```python
from build123d import *

# Parameters (mm, degrees)
SKETCH_1_W          = 17
SKETCH_1_H          = 17
EXTRUDE_1_DEPTH     = 70
SKETCH_2_W          = 12
SKETCH_2_H          = 12
CUT_EXTRUDE_1_DEPTH = 66
SKETCH_3_R          = 1.5
CUT_EXTRUDE_2_DEPTH = 8


with BuildPart() as part:
    # 草图1 → 凸台-拉伸1 (new body)
    with BuildSketch(Plane(origin=(0, 0, 0), x_dir=(1, 0, 0), z_dir=(0, 1, 0))):
        with Locations((8.5, -8.5)):
            Rectangle(SKETCH_1_W, SKETCH_1_H)
    extrude(amount=EXTRUDE_1_DEPTH)

    # 草图2 → 切除-拉伸1 (cut)
    with BuildSketch(Plane(origin=(0, 70, 0), x_dir=(1, 0, 0), z_dir=(0, 1, 0))):
        with Locations((6, -6)):
            Rectangle(SKETCH_2_W, SKETCH_2_H)
    extrude(amount=-CUT_EXTRUDE_1_DEPTH, mode=Mode.SUBTRACT)

    # 草图3 → 切除-拉伸2 (cut)
    with BuildSketch(Plane(origin=(0, 0, 0), x_dir=(-1, 0, 0), z_dir=(0, -1, 0))):
        with Locations(Location((-9.574531369, -2.425468631, 0), (0, 0, 90))):
            Circle(SKETCH_3_R)
        with Locations(Location((-2.425468631, -2.425468631, 0), (0, 0, 90))):
            Circle(SKETCH_3_R)
        with Locations(Location((-9.574531369, -9.574531369, 0), (0, 0, 90))):
            Circle(SKETCH_3_R)
        with Locations(Location((-2.425468631, -9.574531369, 0), (0, 0, 90))):
            Circle(SKETCH_3_R)
    extrude(amount=-CUT_EXTRUDE_2_DEPTH, mode=Mode.SUBTRACT)


solid = part.part
```
The listing builds one solid part. Answer for the finished solid, in the listing's coordinates (mm). A direction names the side the tool comes from. Round coordinates to 2 decimals unless told otherwise and drop trailing zeros. Loops run counter-clockwise (first coordinate to the right, second up) from the corner with the lowest first, then second, coordinate; pieces in that order, holes last. Notation, with made-up numbers: (55.25, 49) - (61.25, 49) arc R15 ccw to (61.25, 64) - close; hole circle Ø7 at (55.5, -27.5). An arc over 180 degrees is marked (long way). Return JSON: item names as keys, results as strings. Group by question number.
1. The mould has two halves that part along Z. Classify faces 3 (the cylindrical face through (1.85, 1.97, 8.19)), 4 (the flat face through (8, 0, 8)), 5 (the flat face through (8, 35, 17)), 6 (the flat face through (12.2, 26.7, 0)): pulls with the +Z half, pulls with the -Z half, needs draft (parallel to the pull), parting line crosses it, or undercut.
2. The part is cut by section C-C on y = 35.5. Determine the outline of the cut face in (x, z).
3. Which of the six approach directions +Z, -Z, +X, -X, +Y, -Y give full straight-line access (tool end or side, diameter ignored) to faces 1 (the flat face through (6, 4, 6)), 2 (the flat face through (17, 35, 9))?
4. The part is cut by section A-A on z = 1.75. Determine the outline of the cut face in (x, y), then the cut area to 3 significant figures.
5. The part is cut by section B-B on x = 3.25. Determine the outline of the cut face in (y, z), then the cut area to 3 significant figures.
6. Each of these flat-tipped pins is pushed along its axis until it touches: P1, Ø6, axis at x = 4.5, y = 13, coming from the -Z side; P2, Ø3.5, axis at x = 8, z = 4.5, coming from the +Y side; P3, Ø3.5, axis at y = 34, z = 6, coming from the -X side. Where does it stop, or does it pass through?
7. Consider probe 1 along X at (y, z) = (66, 10.75); probe 2 along Y at (x, z) = (4.75, 4.25). Determine where each line is inside the solid, lowest interval first.
8. The part is cut by section D-D on z = 6.25. Determine the outline of the cut face in (x, y), then the cut area to 3 significant figures.
Resolved:
{
 "1": {"face 3": "undercut", "face 4": "needs draft", "face 5": "pulls with the +Z half", "face 6": "pulls with the -Z half"},
 "2": {"outline": "(0, 12) - (12, 12) - (12, 0) - (17, 0) - (17, 17) - (0, 17) - close"},
 "3": {"face 1": "-Z, -X, +Y", "face 2": "+Z, -Z, +X, +Y, -Y"},
 "4": {"outline": "(0, 0) - (1.09, 0) - (1.09, 4) - (0, 4) - close; (3.76, 0) - (8.24, 0) - (8.24, 4) - (3.76, 4) - close; (10.91, 0) - (17, 0) - (17, 70) - (12, 70) - (12, 4) - (10.91, 4) - close", "area": "377 mm²"},
 "5": {"outline": "(0, 0) - (4, 0) - (4, 1.17) - (0, 1.17) - close; (0, 3.68) - (4, 3.68) - (4, 8.32) - (0, 8.32) - close; (0, 10.83) - (4, 10.83) - (4, 12) - (70, 12) - (70, 17) - (0, 17) - close", "area": "378 mm²"},
 "6": {"P1": "stops at z = 12", "P2": "stops at y = 4", "P3": "stops at x = 12"},
 "7": {"probe 1": "x = 12 to 17", "probe 2": "y = 0 to 4"},
 "8": {"outline": "(0, 0) - (17, 0) - (17, 70) - (12, 70) - (12, 4) - (0, 4) - close", "area": "398 mm²"}
}
